Geometry check sheet. Reference: the model listing, model coordinates, mm. A direction names the side the tool comes from. Coordinates: 2 decimals unless noted, no trailing zeros. Write each loop counter-clockwise with the first axis right and the second up, starting at its lowest first coordinate (ties: lowest second). Pieces come first, ordered by that corner, then holes.
from build123d import *

# Parameters (mm, degrees)
F0_W     = 20
F0_H     = 20
F0_W_2   = 14
F0_H_2   = 14
F1_DEPTH = 90
F2_R     = 2
F4_D     = 8


with BuildPart() as f1:
    # F0 (on Top) → F1 (new body)
    with BuildSketch(Plane.XY):
        Rectangle(F0_W, F0_H)
        Rectangle(F0_W_2, F0_H_2, mode=Mode.SUBTRACT)
    extrude(amount=F1_DEPTH)

    # F2
    f2_edges = [f1.edges().sort_by_distance(p)[0] for p in [
        (10, -10, 45),
        (10, 10, 45),
        (-10, -10, 45),
        (-10, 10, 45),
    ]]
    fillet(f2_edges, radius=F2_R)

    # F4 (through all)
    with Locations(Plane(origin=(0, 10, 0), x_dir=(-1, 0, 0), z_dir=(0, 1, 0))):
        with Locations((0, 72.4)):
            Hole(F4_D / 2)


solid = f1.part
1. Sectioned sample at D-D, the plane z = 72.4. Record the boundary of the cut face in (x, y), and give its area (3 significant figures).
Computed values:
outline: (-10, -8) arc R2 ccw to (-8, -10) - (-4, -10) - (-4, -7) - (-7, -7) - (-7, 7) - (-4, 7) - (-4, 10) - (-8, 10) arc R2 ccw to (-10, 8) - close; (4, -10) - (8, -10) arc R2 ccw to (10, -8) - (10, 8) arc R2 ccw to (8, 10) - (4, 10) - (4, 7) - (7, 7) - (7, -7) - (4, -7) - close
area: 153 mm2
2. Gauge pin test, flat ends, axial feed: pin 1 Ø10 at (x, y) = (8, 3.5) entering from -Z; pin 2 Ø4 at (x, y) = (-2.5, 3.5) entering from -Z. Record the tip position at first contact, or that the pin passes through.
Computed values:
pin 1: stops at z = 0
pin 2: passes through
3. Access from +Z, -Z, +X, -X, +Y, -Y to the whole of each face (thin tool, end or side, straight path). Record for faces 5 (the flat face through (7, 0, 44)), 6 (the cylindrical face through (9.4, 9.43, 45.63)).
Computed values:
face 5: +Z, -Z
face 6: +Z, -Z, +X, +Y
4. Sectioned sample at C-C, the plane y = -6. Record the boundary of the cut face in (x, z).
Computed values:
outline: (-10, 0) - (-7, 0) - (-7, 90) - (-10, 90) - close; (7, 0) - (10, 0) - (10, 90) - (7, 90) - close
5. Thickness scan on line 1 along X through (y, z) = (0.25, 55); line 2 along Z through (x, y) = (0, -8.8). Record the ranges inside material, lowest first.
Computed values:
line 1: x = -10 to -7, 7 to 10
line 2: z = 0 to 68.4, 76.4 to 90
6. Sectioned sample at B-B, the plane x = 0. Record the boundary of the cut face in (y, z).
Computed values:
outline: (-10, 0) - (-7, 0) - (-7, 68.4) - (-10, 68.4) - close; (-10, 76.4) - (-7, 76.4) - (-7, 90) - (-10, 90) - close; (7, 0) - (10, 0) - (10, 68.4) - (7, 68.4) - close; (7, 76.4) - (10, 76.4) - (10, 90) - (7, 90) - close
7. Draft check along Y on faces 1 (the flat face through (-7, 0, 44)), 2 (the flat face through (0, 7, 44)), 3 (the cylindrical face through (-9.43, -9.4, 45.63)), 4 (the flat face through (10, 0, 44)). Enter one of: released by +Y, released by -Y, zero draft, split by the parting line, or undercut.
Computed values:
face 1: undercut
face 2: undercut
face 3: released by -Y
face 4: zero draft
8. Sectioned sample at A-A, the plane z = 50.5. Record the boundary of the cut face in (x, y), and give its area (3 significant figures).
Computed values:
outline: (-10, -8) arc R2 ccw to (-8, -10) - (8, -10) arc R2 ccw to (10, -8) - (10, 8) arc R2 ccw to (8, 10) - (-8, 10) arc R2 ccw to (-10, 8) - close; hole (-7, -7) - (7, -7) - (7, 7) - (-7, 7) - close
area: 201 mm2
